The figure shows three views and two pictorial views of one solid part (mm, origin at its lowest corner). Answer the questions. A direction names the side the tool comes from. Coordinates: 2 decimals unless noted, no trailing zeros. Loops run counter-clockwise (first coordinate to the right, second up) from the corner with the lowest first, then second, coordinate; pieces in that order, holes last. Notation, with made-up numbers: M -28,89 L 2,89 A23 ccw 2,111 Z; hole C 60,38.25 d6. An arc over 180 degrees is marked long. One line per item, written item: value. Start each with the question number.
1. The part is cut by section B-B (z = 172). Write down the section's boundary in (x, y), then the cut area to 3 significant figures.
2. The part is cut by section A-A (y = 127). Write down the section's boundary in (x, z).
3. The part is cut by section C-C (x = 176). Write down the section's boundary in (y, z).
4. For the marked faces 1 and 2, determine the directions among +Z, -Z, +X, -X, +Y, -Y from which every point of the face is accessible in a straight line to the end or side of a thin tool.
5. A flat-ended cylindrical pin translates along its axis: pin 1 (10 mm diameter, centred on x = 210.5, z = 78.5, fed in from -Y). Find the tip coordinate at first contact, or state that the pin passes through.
6. Determine the mould class of the marked faces 3, 4, 5 and 6 for opening direction X: +X half, -X half, draft (parallel to the pull), parting line (faces both ways), or undercut.
7. Consider probe 1 along Z at (x, y) = (123.5, 235); probe 2 along X at (y, z) = (87, 199); probe 3 along Z at (x, y) = (120, 150) (1 decimal). Determine where each line is inside the solid, lowest interval first.
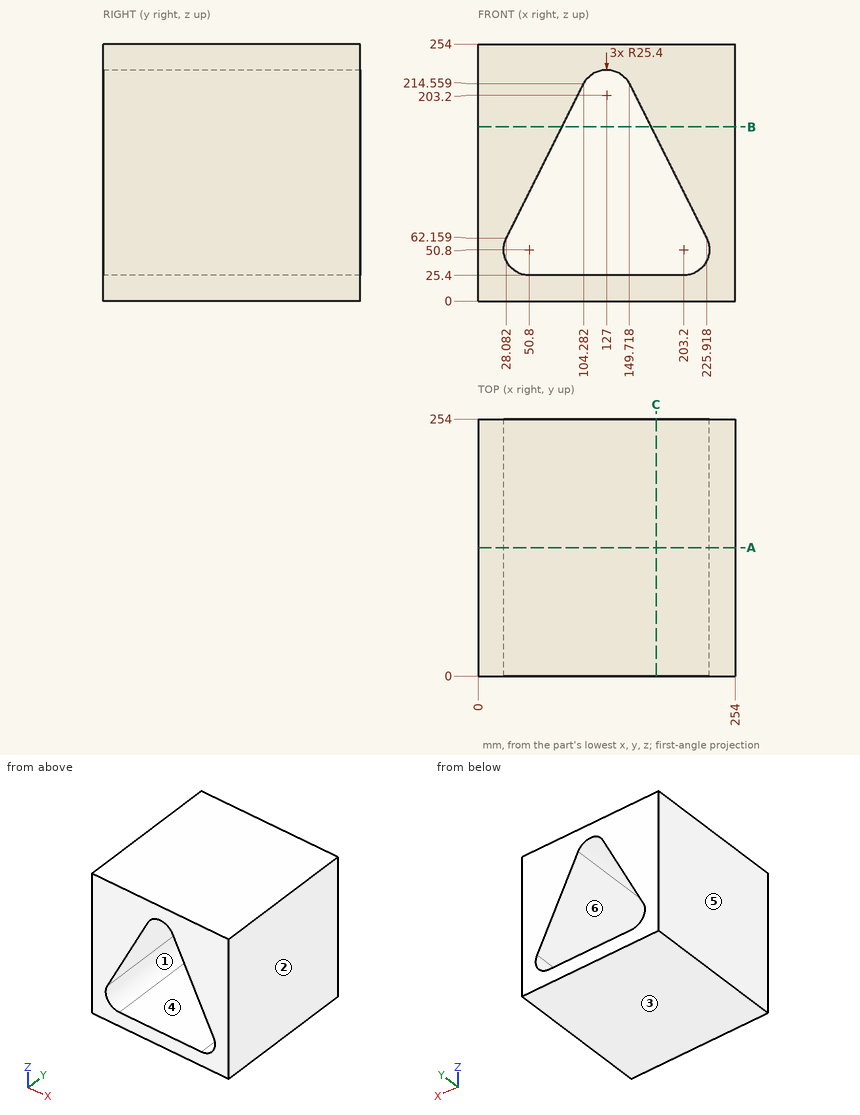
Answer block:
1. outline: M 0,0 L 83,0 L 83,254 L 0,254 Z; M 171,0 L 254,0 L 254,254 L 171,254 Z
1. area: 42,200 mm2
2. outline: M 0,0 L 254,0 L 254,254 L 0,254 Z; hole M 28.08,62.16 A25.4 ccw 50.8,25.4 L 203.2,25.4 A25.4 ccw 225.92,62.16 L 149.72,214.56 A25.4 ccw 104.28,214.56 Z
3. outline: M 0,0 L 254,0 L 254,25.4 L 0,25.4 Z; M 0,162 L 254,162 L 254,254 L 0,254 Z
4. face 1: +Y, -Y
4. face 2: +Z, -Z, +X, +Y, -Y
5. pin 1: passes through
6. face 3: draft
6. face 4: undercut
6. face 5: -X half
6. face 6: undercut
7. probe 1: z = 0 to 25.4, 228.36 to 254
7. probe 2: x = 0 to 96.5, 157.5 to 254
7. probe 3: z = 0 to 25.4, 227.6 to 254
